For this review, take the finished solid that the model builds, in its own axes (mm). A direction names the side the tool comes from. Give positions to 0.01 mm unless a question says otherwise; leave off trailing zeros. Order: outer loops, then holes, each group sorted by start corner. A loop starts at its lowest first (then second) coordinate and runs counter-clockwise, first axis right, second up. Notation, with made-up numbers: (15.25, 46.25) - (24.25, 46.25) arc R19 cw to (24.25, 75.25) - close; hole circle Ø2 at (76, 35). An arc over 180 degrees is marked (long way). Use a Markdown table: item, result. Add a question column.
1) Mouldability with a two-part tool opening along Z and no side actions: class faces 1 (the face through (5, 10, 0)), 2 (the face through (0, 7, -7.5)), 3 (the face through (-7.5, 7, 0)) as released by +Z, released by -Z, zero draft, split by the parting line, or undercut.
2) Wall thickness on L1, parallel to Y at x = -3, z = -1.25; L2, parallel to X at y = 7.5, z = -1; L3, parallel to Z at x = 0, y = 9.25: over which ranges is each line inside the solid? List them lowest first.
3) Machinability: for faces 4 (the face through (5, 13, 2.202)), 5 (the face through (0, 7, 7.5)), 6 (the face through (-5, 10, 0)), which of the approach directions +Z, -Z, +X, -X, +Y, -Y give a long, thin tool a straight path to every point of the face, cutting with its end or side? Answer none if there is none.
4) We need section B-B on z = 0. Write out the cut boundary in (x, y).
5) We need section A-A on x = 0. Write out the cut boundary in (y, z).
6) We need section C-C on y = 6.5. Write out the cut boundary in (x, z).
7) We need section D-D on y = 11.25. Write out the cut boundary in (x, z).
8) Clearance check with a flat-ended pin moving along its axis: P1, Ø1.5, axis at x = -5.5, z = 0.5, coming from the -Y side. State where the tip first meets the part, or that it passes through.
```python
from build123d import *

# Parameters (mm, degrees)
ESQUISSE1_W             = 15
ESQUISSE1_H             = 15
ESQUISSE1_R             = 3
BOSS_EXTRU_1_DEPTH      = 15
ESQUISSE2_W             = 4.404326356
ESQUISSE2_H             = 1.565605919
ENL_V_MAT_EXTRU_1_DEPTH = 15
ESQUISSE3_R             = 1.5
ENL_V_MAT_EXTRU_2_DEPTH = 10


with BuildPart() as part:
    # Esquisse1 → Boss.-Extru.1 (new body)
    with BuildSketch(Plane(origin=(0, 0, 0), x_dir=(1, 0, 0), z_dir=(0, 1, 0))):
        Rectangle(ESQUISSE1_W, ESQUISSE1_H)
        Circle(ESQUISSE1_R, mode=Mode.SUBTRACT)
    extrude(amount=BOSS_EXTRU_1_DEPTH)

    # Esquisse2 → Enlèv. mat.-Extru.1 (cut)
    with BuildSketch(Plane(origin=(7.5, 0, 0), x_dir=(0, 0, -1), z_dir=(1, 0, 0))):
        with Locations((0, 12.899904082)):
            Rectangle(ESQUISSE2_W, ESQUISSE2_H)
    extrude(amount=-ENL_V_MAT_EXTRU_1_DEPTH, mode=Mode.SUBTRACT)

    # Esquisse3 → Enlèv. mat.-Extru.2 (cut)
    with BuildSketch(Plane.XZ):
        with Locations((5, 0)):
            Circle(ESQUISSE3_R)
        with Locations((-5, 0)):
            Circle(ESQUISSE3_R)
    extrude(amount=-ENL_V_MAT_EXTRU_2_DEPTH, mode=Mode.SUBTRACT)


solid = part.part
```
Checked values:
| question | item | result |
|---|---|---|
| 1 | face 1 | undercut |
| 1 | face 2 | released by -Z |
| 1 | face 3 | zero draft |
| 2 | L1 | 0 to 12.12, 13.68 to 15 |
| 2 | L2 | -7.5 to -6.12, -3.88 to -2.83, 2.83 to 3.88, 6.12 to 7.5 |
| 2 | L3 | -7.5 to -3, 3 to 7.5 |
| 3 | face 4 | +X, -X |
| 3 | face 5 | +Z, +X, -X, +Y, -Y |
| 3 | face 6 | -Y |
| 4 | outline | (-7.5, 0) - (-6.5, 0) - (-6.5, 10) - (-3.5, 10) - (-3.5, 0) - (-3, 0) - (-3, 12.12) - (-7.5, 12.12) - close; (-7.5, 13.68) - (-3, 13.68) - (-3, 15) - (-7.5, 15) - close; (3, 0) - (3.5, 0) - (3.5, 10) - (6.5, 10) - (6.5, 0) - (7.5, 0) - (7.5, 12.12) - (3, 12.12) - close; (3, 13.68) - (7.5, 13.68) - (7.5, 15) - (3, 15) - close |
| 5 | outline | (0, -7.5) - (15, -7.5) - (15, -3) - (0, -3) - close; (0, 3) - (15, 3) - (15, 7.5) - (0, 7.5) - close |
| 6 | outline | (-7.5, -7.5) - (7.5, -7.5) - (7.5, 7.5) - (-7.5, 7.5) - close; hole circle Ø3 at (-5, 0); hole circle Ø6 at (0, 0); hole circle Ø3 at (5, 0) |
| 7 | outline | (-7.5, -7.5) - (7.5, -7.5) - (7.5, 7.5) - (-7.5, 7.5) - close; hole circle Ø6 at (0, 0) |
| 8 | P1 | y = 10 |
